Autodesk Inventor part; units mm, degrees
ref_plane "Work Plane1" through (-19.467767, 1.0375, -4.375) normal (0, 0, -1) x (0, 1, 0)
ref_plane "YZ Plane" through (0, 0, 0) normal (1, 0, 0) x (0, 1, 0)
ref_plane "XZ Plane" through (0, 0, 0) normal (0, 1, 0) x (-1, 0, 0)
sketch "Sketch1" plane through (0, 0, 0) normal (0, 0, 1) x (1, 0, 0)
  circle A0 centre (151.367767, 26.667767) radius 7
  circle A1 centre (151.367767, 26.667767) radius 6.965
  circle A2 centre (151.367767, 26.667767) radius 6.09
  point P0 (0, 0)
  dimension "d0" = 0.035
  dimension "d2" = 0.875
ref_plane "Work Plane1" through (-19.467767, 1.0375, -4.375) normal (0, 0, -1) x (0, 1, 0)
sketch "Sketch1 outline for Extrusion1" plane through (0, 0, 0) normal (0, 0, 1) x (1, 0, 0)
  circle A0 centre (151.367767, 26.667767) radius 6.965
  circle A1 centre (151.367767, 26.667767) radius 6.09
extrude "Extrusion1" add sketch "Sketch1 outline for Extrusion1" along normal blind 2.5 from surface at -4.375
sketch "Sketch2" plane through (151.367767, 26.667767, -4.375) normal (0, 0, -1) x (-1, 0, 0)
  circle A0 centre (0, 0) radius 6.965
  circle A1 centre (0, 0) radius 6.09
  circle A2 centre (0, 0) radius 7.09
  circle A3 centre (0, 0) radius 9.09
  point P0 (151.367767, -26.667767)
  dimension "d5" = 0.125
  dimension "d6" = 2
extrude "Extrusion2" add sketch "Sketch2" along normal blind 1.25 contours A0 | A2 | A3
properties part number "Half Inch Lense Holder Cover (V5)"
CAD build for the part. Positions are in the model's coordinates, mm. Round coordinates to 2 decimals unless told otherwise and drop trailing zeros. Write each loop counter-clockwise with the first axis right and the second up, starting at its lowest first coordinate (ties: lowest second). Pieces come first, ordered by that corner, then holes. Notation, with made-up numbers: (5, -22.5) - (51, -22.5) arc R20 ccw to (51, -18.5) - close; hole circle Ø3 at (4, 88.5). An arc over 180 degrees is marked (long way). Return JSON: item names as keys, results as strings. Group by question number.
Item 1: Flat gauge pins, fed straight in: pin 1 Ø2 at (x, z) = (156.5, -4.5) entering from +Y; pin 2 Ø5.5 at (x, y) = (156, 24.5) entering from +Z (3 decimals); pin 3 Ø1.5 at (y, z) = (20.5, -4.5) entering from +X. Where does each tip first touch, or does it go through?
Item 2: Band-saw the part on B-B on y = 27.5. List the corners of the cut face in (x, z) (3 decimals).
Item 3: Band-saw the part on A-A on x = 148.25. List the corners of the cut face in (y, z) (3 decimals).
Item 4: Band-saw the part on D-D on z = -4.85. List the corners of the cut face in (x, y).
Item 5: Mould opens along Z. For faces 1 (the face through (142.698, 23.937, -4.991)), 2 (the face through (145, 25, -5.625)), 3 (the face through (154, 21, -1.875)) say: +Z half, -Z half, draft (parallel to the pull), parting line (faces both ways), or undercut.
Item 6: Band-saw the part on C-C on y = 33. List the corners of the cut face in (x, z) (3 decimals), plus the area to 3 significant figures.
Item 7: Probe probe 1 along Y at (x, z) = (151.25, -4.05); probe 2 along Z at (x, y) = (145.5, 31.75) (3 decimals); probe 3 along Y at (x, z) = (156.5, -3.8). List the from-to ranges inside material, lowest first.
Resolved:
{
 "1": {"pin 1": "stops at y = 34.76", "pin 2": "stops at z = -1.875", "pin 3": "stops at x = 158.67"},
 "2": {"outline": "(142.316, -5.625) - (145.335, -5.625) - (145.335, -1.875) - (144.453, -1.875) - (144.453, -4.375) - (142.316, -4.375) - close; (157.401, -5.625) - (160.42, -5.625) - (160.42, -4.375) - (158.283, -4.375) - (158.283, -1.875) - (157.401, -1.875) - close"},
 "3": {"outline": "(18.129, -5.625) - (21.436, -5.625) - (21.436, -1.875) - (20.44, -1.875) - (20.44, -4.375) - (18.129, -4.375) - close; (31.899, -5.625) - (35.206, -5.625) - (35.206, -4.375) - (32.896, -4.375) - (32.896, -1.875) - (31.899, -1.875) - close"},
 "4": {"outline": "circle Ø18.18 at (151.37, 26.67); hole circle Ø12.18 at (151.37, 26.67)"},
 "5": {"face 1": "draft", "face 2": "-Z half", "face 3": "+Z half"},
 "6": {"outline": "(144.846, -5.625) - (157.889, -5.625) - (157.889, -4.375) - (154.268, -4.375) - (154.268, -1.875) - (148.467, -1.875) - (148.467, -4.375) - (144.846, -4.375) - close", "area": "30.8 mm²"},
 "7": {"probe 1": "y = 19.7 to 20.58, 32.76 to 33.63", "probe 2": "z = -5.625 to -4.375", "probe 3": "y = 21.96 to 23.39, 29.95 to 31.38"}
}
